Design review of the part built by this model. Coordinates are the model's own, in mm. A direction names the side the tool comes from. Coordinates: 2 decimals unless noted, no trailing zeros. Loops run counter-clockwise (first coordinate to the right, second up) from the corner with the lowest first, then second, coordinate; pieces in that order, holes last. Notation, with made-up numbers: (47, -6.5) - (83, -6.5) arc R24 ccw to (83, 30.5) - close; hole circle Ø11 at (8.5, 59.5). An arc over 180 degrees is marked (long way). Answer in a Markdown table with one row per item. Add a question column.
(1) We need section B-B, the plane x = 0. Write out the cut boundary in (y, z), plus the area to 3 significant figures.
(2) For faces 1 (the face through (-12, 25, 1)), 2 (the face through (12.465, 12.325, -56.133)), list the 3-axis set-ups (+Z, -Z, +X, -X, +Y, -Y) from which the entire face can be reached by the end or side of a thin tool; tool diameter is ignored.
(3) The part is to be moulded in two halves that separate along X. For faces 3 (the face through (-3.78, 4.72, -2.9)), 4 (the face through (-17, 0, -55.2)), 5 (the face through (-9.764, -7.395, 74.362)), say which applies: released by +X, released by -X, zero draft, split by the parting line, or undercut.
(4) To check wall thickness, follow L1, parallel to Z at x = 0, y = 3; L2, parallel to Z at x = 0, y = -0.5; L3, parallel to Y at x = 69.5, z = 3.5. State the ranges of each line that lie inside material, in increasing order. Write a range as [from, to].
(5) We need section A-A, the plane z = 0. Write out the cut boundary in (x, y), plus the area to 3 significant figures.
(6) Clearance check with flat-ended pins moving along their axes: pin 1 (1.5 mm diameter, centred on y = -4.5, z = 54, fed in from -X); pin 2 (1 mm diameter, centred on y = 15.5, z = -22, fed in from -X); pin 3 (5 mm diameter, centred on y = 12, z = -51, fed in from -X). State where each tip first meets the part, or that it passes through.
(7) We need section D-D, the plane z = 42. Write out the cut boundary in (x, y), plus the area to 3 significant figures.
(8) We need section C-C, the plane y = 18. Write out the cut boundary in (x, z) (1 decimal).
from build123d import *

# Parameters (mm, degrees)
F0_R     = 75
F1_DEPTH = 15
F2_R     = 57.5
F3_DEPTH = 25
F4_R     = 4.7625
F5_DEPTH = 40.001


with BuildPart() as f1:
    # F0 (on Front) → F1 (new body)
    with BuildSketch(Plane.XZ):
        Circle(F0_R)
    extrude(amount=F1_DEPTH)

    # F2 (on face) → F3 (join)
    with BuildSketch(Plane(origin=(0, 0, 0), x_dir=(-1, 0, 0), z_dir=(0, 1, 0))):
        Circle(F2_R)
    extrude(amount=F3_DEPTH)

    # F4 (on face) → F5 (cut, through all)
    with BuildSketch(Plane.XZ.offset(15)):
        Circle(F4_R)
    extrude(amount=-F5_DEPTH, mode=Mode.SUBTRACT)


solid = f1.part
Responses:
| question | item | result |
|---|---|---|
| 1 | outline | (-15, -75) - (0, -75) - (0, -57.5) - (25, -57.5) - (25, -4.76) - (-15, -4.76) - close; (-15, 4.76) - (25, 4.76) - (25, 57.5) - (0, 57.5) - (0, 75) - (-15, 75) - close |
| 1 | area | 4,740 mm2 |
| 2 | face 1 | +Z, -Z, +X, -X, +Y |
| 2 | face 2 | +Y |
| 3 | face 3 | undercut |
| 3 | face 4 | zero draft |
| 3 | face 5 | split by the parting line |
| 4 | L1 | z = [-57.5, -4.76], [4.76, 57.5] |
| 4 | L2 | z = [-75, -4.76], [4.76, 75] |
| 4 | L3 | y = [-15, 0] |
| 5 | outline | (-75, -15) - (-4.76, -15) - (-4.76, 25) - (-57.5, 25) - (-57.5, 0) - (-75, 0) - close; (4.76, -15) - (75, -15) - (75, 0) - (57.5, 0) - (57.5, 25) - (4.76, 25) - close |
| 5 | area | 4,740 mm2 |
| 6 | pin 1 | stops at x = -52.82 |
| 6 | pin 2 | stops at x = -53.33 |
| 6 | pin 3 | stops at x = -30.89 |
| 7 | outline | (-62.14, -15) - (62.14, -15) - (62.14, 0) - (39.27, 0) - (39.27, 25) - (-39.27, 25) - (-39.27, 0) - (-62.14, 0) - close |
| 7 | area | 3,830 mm2 |
| 8 | outline | circle Ø115 at (0, 0); hole circle Ø9.5 at (0, 0) |
